from build123d import *

# Parameters (mm, degrees)
SKETCH1_W           = 76
SKETCH1_H           = 21
BOSS_EXTRUDE1_DEPTH = 4
SKETCH2_W           = 76
SKETCH2_H           = 3.8
BOSS_EXTRUDE2_DEPTH = 26
SKETCH3_W           = 62
SKETCH3_H           = 22
BOSS_EXTRUDE3_DEPTH = 15.7
CHAMFER2_SIZE       = 2
SKETCH4_W           = 55.8
SKETCH4_H           = 8.6
CUT_EXTRUDE1_DEPTH  = 0.6
CUT_EXTRUDE2_DEPTH  = 46.14698218
SKETCH6_W           = 8
SKETCH6_H           = 4
CUT_EXTRUDE3_DEPTH  = 19.7
SKETCH7_W           = 58
SKETCH7_H           = 15.4
CUT_EXTRUDE4_DEPTH  = 13.7
CUT_EXTRUDE5_DEPTH  = 13.7
LPATTERN1_COUNT     = 3
LPATTERN1_PITCH     = 25.8
BOSS_EXTRUDE4_REACH = 52.606
SKETCH9_W           = 1.9
SKETCH9_H           = 15.4
CUT_EXTRUDE6_REACH  = 53.418
CUT_EXTRUDE7_REACH  = 76.48
SKETCH12_W          = 1.2
SKETCH12_H          = 3.8
CUT_EXTRUDE8_DEPTH  = 11.9
CUT_EXTRUDE9_REACH  = 50.647
SKETCH13_R          = 2.5


with BuildPart() as part:
    # Sketch1 → Boss-Extrude1 (new body)
    with BuildSketch(Plane(origin=(0, 0, 0), x_dir=(1, 0, 0), z_dir=(0, 1, 0))):
        Rectangle(SKETCH1_W, SKETCH1_H)
    extrude(amount=BOSS_EXTRUDE1_DEPTH)

    # Sketch2 → Boss-Extrude2 (add)
    with BuildSketch(Plane(origin=(0, 0, 0), x_dir=(1, 0, 0), z_dir=(0, 1, 0))):
        with Locations((0, -8.6)):
            Rectangle(SKETCH2_W, SKETCH2_H)
    extrude(amount=BOSS_EXTRUDE2_DEPTH)

    # Sketch3 → Boss-Extrude3 (add)
    with BuildSketch(Plane(origin=(0, 0, 10.5), x_dir=(-1, 0, 0), z_dir=(0, 0, -1))):
        with Locations((0, 15)):
            Rectangle(SKETCH3_W, SKETCH3_H)
    extrude(amount=BOSS_EXTRUDE3_DEPTH)

    # Chamfer2
    chamfer2_edges = [part.edges().sort_by_distance(p)[0] for p in [
        (-38, 2, -10.5),
        (38, 2, -10.5),
    ]]
    chamfer(chamfer2_edges, length=CHAMFER2_SIZE)

    # Sketch4 → Cut-Extrude1 (cut)
    with BuildSketch(Plane(origin=(0, 26, 0), x_dir=(1, 0, 0), z_dir=(0, 1, 0))):
        with Locations((0, -1.9)):
            Rectangle(SKETCH4_W, SKETCH4_H)
    extrude(amount=-CUT_EXTRUDE1_DEPTH, mode=Mode.SUBTRACT)

    # Sketch5 → Cut-Extrude2 (cut, through all)
    with BuildSketch(Plane(origin=(0, 4, 0), x_dir=(1, 0, 0), z_dir=(0, 1, 0))):
        with BuildLine():
            Line((-32, 2.7), (-32, -3.3))
            ThreePointArc((-32, -3.3), (-34, -5.3), (-36, -3.3))
            Line((-36, -3.3), (-36, 2.7))
            ThreePointArc((-36, 2.7), (-34, 4.7), (-32, 2.7))
        make_face()
        with BuildLine():
            Line((32, 2.7), (32, -3.3))
            ThreePointArc((32, -3.3), (34, -5.3), (36, -3.3))
            Line((36, -3.3), (36, 2.7))
            ThreePointArc((36, 2.7), (34, 4.7), (32, 2.7))
        make_face()
    extrude(amount=-CUT_EXTRUDE2_DEPTH, mode=Mode.SUBTRACT)

    # Sketch6 → Cut-Extrude3 (cut)
    with BuildSketch(Plane(origin=(0, 0, -10.5), x_dir=(-1, 0, 0), z_dir=(0, 0, -1))):
        with Locations((-12.75, 3.1)):
            Rectangle(SKETCH6_W, SKETCH6_H)
        with Locations((12.75, 3.1)):
            Rectangle(SKETCH6_W, SKETCH6_H)
    extrude(amount=-CUT_EXTRUDE3_DEPTH, mode=Mode.SUBTRACT)

    # Sketch7 → Cut-Extrude4 (cut)
    with BuildSketch(Plane.XY.offset(10.5)):
        with Locations((0, 13)):
            Rectangle(SKETCH7_W, SKETCH7_H)
    extrude(amount=-CUT_EXTRUDE4_DEPTH, mode=Mode.SUBTRACT)

    # Sketch8 → Cut-Extrude5 (cut)
    with BuildSketch(Plane.XY.offset(10.5)):
        with BuildLine():
            Line((-29, 23), (-29, 3))
            ThreePointArc((-29, 3), (-25.8, 2.15), (-22.6, 3))
            Line((-22.6, 3), (-22.6, 23))
            ThreePointArc((-22.6, 23), (-25.8, 23.85), (-29, 23))
        make_face()
    cut_extrude5 = extrude(amount=-CUT_EXTRUDE5_DEPTH, mode=Mode.SUBTRACT)

    # LPattern1: Cut-Extrude5 ×3
    with Locations(*[(i * LPATTERN1_PITCH, 0, 0) for i in range(1, LPATTERN1_COUNT)]):
        add(cut_extrude5, mode=Mode.SUBTRACT)

    # Sketch9 → Boss-Extrude4 (add, up to next)
    with BuildSketch(Plane.XY.offset(10.5), mode=Mode.PRIVATE) as boss_extrude4_sk1:
        with Locations((-4.15, 13)):
            Rectangle(SKETCH9_W, SKETCH9_H)
    boss_extrude4_tool1 = extrude(boss_extrude4_sk1.sketch, amount=-BOSS_EXTRUDE4_REACH, mode=Mode.PRIVATE) - part.part
    # Sketch9 → Boss-Extrude4 (add, up to next)
    with BuildSketch(Plane.XY.offset(10.5), mode=Mode.PRIVATE) as boss_extrude4_sk2:
        with Locations((4.15, 13)):
            Rectangle(SKETCH9_W, SKETCH9_H)
    boss_extrude4_tool2 = extrude(boss_extrude4_sk2.sketch, amount=-BOSS_EXTRUDE4_REACH, mode=Mode.PRIVATE) - part.part
    add(boss_extrude4_tool1.solids().sort_by_distance((-4.15, 13, 10.5))[0])
    add(boss_extrude4_tool2.solids().sort_by_distance((4.15, 13, 10.5))[0])

    # Cut-Extrude6: up to this face of the body (flat: up to its plane)
    cut_extrude6_end = Plane(part.part.faces().sort_by_distance((5.1, 13, 3.65))[0])
    # Sketch10 → Cut-Extrude6 (cut, up to the picked face)
    with BuildSketch(Plane.ZY.offset(5.1), mode=Mode.PRIVATE) as cut_extrude6_sk1:
        with BuildLine():
            Line((10.5, 15.25), (1.75, 15.25))
            ThreePointArc((1.75, 15.25), (-0.5, 13), (1.75, 10.75))
            Line((1.75, 10.75), (10.5, 10.75))
            Line((10.5, 10.75), (10.5, 15.25))
        make_face()
    cut_extrude6_tool1 = split(extrude(cut_extrude6_sk1.sketch, amount=-CUT_EXTRUDE6_REACH, mode=Mode.PRIVATE), bisect_by=cut_extrude6_end, keep=Keep.BOTH, mode=Mode.PRIVATE)
    add(cut_extrude6_tool1.solids().sort_by(Axis((-5.1, 13, 5.229437), (1, 0, 0)))[0], mode=Mode.SUBTRACT)

    # Sketch11 → Cut-Extrude7 (cut, up to next)
    with BuildSketch(Plane.ZY.offset(31), mode=Mode.PRIVATE) as cut_extrude7_sk1:
        Polygon((1.5, 17.5), (-2.5, 15.190598923), (-2.5, 10.57179677), (1.5, 8.262395693), (5.5, 10.57179677), (5.5, 15.190598923), align=None)
    cut_extrude7_tool1 = extrude(cut_extrude7_sk1.sketch, amount=-CUT_EXTRUDE7_REACH, mode=Mode.PRIVATE) & part.part
    cut_extrude7 = cut_extrude7_tool1.solids().sort_by_distance((-31, 12.881198, 1.5))[0]
    add(cut_extrude7, mode=Mode.SUBTRACT)

    # Mirror1: Cut-Extrude7 across plane
    add(cut_extrude7.mirror(Plane(origin=(0, 0, 0), x_dir=(0, 0, 1), z_dir=(1, 0, 0))), mode=Mode.SUBTRACT)

    # Sketch12 → Cut-Extrude8 (cut)
    with BuildSketch(Plane(origin=(0, 0, -5.2), x_dir=(-1, 0, 0), z_dir=(0, 0, -1))):
        with Locations((-30.4, 5.9)):
            Rectangle(SKETCH12_W, SKETCH12_H)
        with Locations((30.4, 5.9)):
            Rectangle(SKETCH12_W, SKETCH12_H)
    extrude(amount=-CUT_EXTRUDE8_DEPTH, mode=Mode.SUBTRACT)

    # Sketch13 → Cut-Extrude9 (cut, up to next)
    with BuildSketch(Plane(origin=(0, 0, -5.2), x_dir=(-1, 0, 0), z_dir=(0, 0, -1)), mode=Mode.PRIVATE) as cut_extrude9_sk1:
        with Locations((-25.5, 18.1)):
            Circle(SKETCH13_R)
    cut_extrude9_tool1 = extrude(cut_extrude9_sk1.sketch, amount=-CUT_EXTRUDE9_REACH, mode=Mode.PRIVATE) & part.part
    # Sketch13 → Cut-Extrude9 (cut, up to next)
    with BuildSketch(Plane(origin=(0, 0, -5.2), x_dir=(-1, 0, 0), z_dir=(0, 0, -1)), mode=Mode.PRIVATE) as cut_extrude9_sk2:
        with Locations((0.3, 18.1)):
            Circle(SKETCH13_R)
    cut_extrude9_tool2 = extrude(cut_extrude9_sk2.sketch, amount=-CUT_EXTRUDE9_REACH, mode=Mode.PRIVATE) & part.part
    # Sketch13 → Cut-Extrude9 (cut, up to next)
    with BuildSketch(Plane(origin=(0, 0, -5.2), x_dir=(-1, 0, 0), z_dir=(0, 0, -1)), mode=Mode.PRIVATE) as cut_extrude9_sk3:
        with Locations((26.1, 18.1)):
            Circle(SKETCH13_R)
    cut_extrude9_tool3 = extrude(cut_extrude9_sk3.sketch, amount=-CUT_EXTRUDE9_REACH, mode=Mode.PRIVATE) & part.part
    # Sketch13 → Cut-Extrude9 (cut, up to next)
    with BuildSketch(Plane(origin=(0, 0, -5.2), x_dir=(-1, 0, 0), z_dir=(0, 0, -1)), mode=Mode.PRIVATE) as cut_extrude9_sk4:
        with Locations((0.3, 8.1)):
            Circle(SKETCH13_R)
    cut_extrude9_tool4 = extrude(cut_extrude9_sk4.sketch, amount=-CUT_EXTRUDE9_REACH, mode=Mode.PRIVATE) & part.part
    # Sketch13 → Cut-Extrude9 (cut, up to next)
    with BuildSketch(Plane(origin=(0, 0, -5.2), x_dir=(-1, 0, 0), z_dir=(0, 0, -1)), mode=Mode.PRIVATE) as cut_extrude9_sk5:
        with Locations((26.1, 8.1)):
            Circle(SKETCH13_R)
    cut_extrude9_tool5 = extrude(cut_extrude9_sk5.sketch, amount=-CUT_EXTRUDE9_REACH, mode=Mode.PRIVATE) & part.part
    # Sketch13 → Cut-Extrude9 (cut, up to next)
    with BuildSketch(Plane(origin=(0, 0, -5.2), x_dir=(-1, 0, 0), z_dir=(0, 0, -1)), mode=Mode.PRIVATE) as cut_extrude9_sk6:
        with Locations((-25.5, 8.1)):
            Circle(SKETCH13_R)
    cut_extrude9_tool6 = extrude(cut_extrude9_sk6.sketch, amount=-CUT_EXTRUDE9_REACH, mode=Mode.PRIVATE) & part.part
    add(cut_extrude9_tool1.solids().sort_by_distance((25.5, 18.1, -5.2))[0], mode=Mode.SUBTRACT)
    add(cut_extrude9_tool2.solids().sort_by_distance((-0.3, 18.1, -5.2))[0], mode=Mode.SUBTRACT)
    add(cut_extrude9_tool3.solids().sort_by_distance((-26.1, 18.1, -5.2))[0], mode=Mode.SUBTRACT)
    add(cut_extrude9_tool4.solids().sort_by_distance((-0.3, 8.1, -5.2))[0], mode=Mode.SUBTRACT)
    add(cut_extrude9_tool5.solids().sort_by_distance((-26.1, 8.1, -5.2))[0], mode=Mode.SUBTRACT)
    add(cut_extrude9_tool6.solids().sort_by_distance((25.5, 8.1, -5.2))[0], mode=Mode.SUBTRACT)


solid = part.part
Geometry: final body of the model. Coordinates: model frame, mm. A direction names the side the tool comes from. Round coordinates to 2 decimals unless told otherwise and drop trailing zeros. Loops run counter-clockwise (first coordinate to the right, second up) from the corner with the lowest first, then second, coordinate; pieces in that order, holes last. Notation, with made-up numbers: M 37.5,85.5 L 49.5,85.5 A26 ccw 49.5,122.5 Z; hole C -20,68 d5. An arc over 180 degrees is marked long. One line per question, with ' | ' between items.
(1) Cut plane D-D on z = 8.5. Give the number of separate pieces and of enclosed holes in the cut face, plus the area to 3 significant figures.
Check result:
separate pieces: 1 | enclosed holes: 3 | area: 950 mm2
(2) Cut plane C-C on x = -25. Return the cut outline in (y, z) (3 decimals), plus the area to 3 significant figures.
Check result:
outline: M 0,-10.5 L 4,-10.5 L 4,-5.2 L 5.855,-5.2 L 5.855,-3.2 L 2.2,-3.2 L 2.2,10.5 L 0,10.5 Z; M 10.345,-5.2 L 15.855,-5.2 L 15.855,-3.2 L 10.345,-3.2 Z; M 20.345,-5.2 L 26,-5.2 L 26,-2.4 L 25.4,-2.4 L 25.4,6.2 L 26,6.2 L 26,10.5 L 23.8,10.5 L 23.8,-3.2 L 20.345,-3.2 Z | area: 110 mm2
(3) Cut plane A-A on x = 34. Return the cut outline in (y, z), plus the area to 3 significant figures.
Check result:
outline: M 0,-10.5 L 4,-10.5 L 4,-4.7 L 0,-4.7 Z; M 0,5.3 L 4,5.3 L 4,6.7 L 26,6.7 L 26,10.5 L 0,10.5 Z | area: 128 mm2
(4) Access query for faces 1 (the flat face through (-14, 20.7, 4)), 2 (the flat face through (0, 25.4, 2)), 3 (the flat face through (30.01, 16.33, 3.53)), 4 (the flat face through (31, 19, 1)). Directions: +Z, -Z, +X, -X, +Y, -Y. A direction counts if a zero-diameter tool reaches every point of the face in a straight line with its end or side. Return the directions, or none.
Check result:
face 1: +Z | face 2: +Y | face 3: +X | face 4: -Z, +X, +Y
(5) Material intervals for line 1 along Y through (x, z) = (-26.1, -4.55); line 2 along X through (y, z) = (21.25, 4); line 3 along X through (y, z) = (5.5, 3), sorted ascending. Write a range as from..to.
Check result:
line 1: y = 0..5.6, 10.6..15.6, 20.6..26 | line 2: x = -31..-29, -22.6..-3.2, 3.2..22.6, 29..31 | line 3: x = -29.8..-29, -5.1..-3.2, 3.2..5.1, 29..29.8
(6) Cut plane B-B on y = 13.5. Return the cut outline in (x, z).
Check result:
outline: M -38,6.7 L -31,6.7 L -31,5.5 L -29,5.5 L -29,10.5 L -38,10.5 Z; M -31,-5.2 L 31,-5.2 L 31,-2.5 L 29,-2.5 L 29,-3.2 L 5.1,-3.2 L 5.1,-0.44 L 3.2,-0.44 L 3.2,-3.2 L -3.2,-3.2 L -3.2,-0.44 L -5.1,-0.44 L -5.1,-3.2 L -29,-3.2 L -29,-2.5 L -31,-2.5 Z; M 29,5.5 L 31,5.5 L 31,6.7 L 38,6.7 L 38,10.5 L 29,10.5 Z
(7) Pull-direction query (Z, two-part tool) for faces 5 (the flat face through (-29, 13, 7)), 6 (the flat face through (-37, 2, -9.5)), 7 (the flat face through (-30.01, 16.33, 3.53)); classes: +Z half, -Z half, draft (parallel to the pull), parting line (faces both ways), or undercut.
Check result:
face 5: draft | face 6: -Z half | face 7: undercut
(8) Contact query for flat-ended pins moving along their axis: P1, Ø6.5, axis at x = 15, y = 15.5, coming from the +Z side; P2, Ø2, axis at x = 16, y = 10.5, coming from the -Z side; P3, Ø0.5, axis at y = 25.5, z = 3.5, coming from the +X side. Output: stop coordinate, or through.
Check result:
P1: stops at z = -3.2 | P2: stops at z = -5.2 | P3: stops at x = 31
